```python
from build123d import *

# Parameters (mm, degrees)
SKETCH_3_W                = 201
SKETCH_3_H                = 142
EXTRUDE_2_DEPTH           = 5
SKETCH_4_W                = 171
SKETCH_4_H                = 112
CUT_EXTRUDE_1_DEPTH       = 2.5
SKETCH_5_W                = 50
SKETCH_5_H                = 20
CUT_EXTRUDE_6_DEPTH       = 15
SKETCH_6_R                = 1.2
CUT_EXTRUDE_7_DEPTH       = 3
CUT_EXTRUDE_8_REACH       = 215.23
HOLE_WIZARD_1_D           = 2.4
HOLE_WIZARD_1_CSINK_D     = 4.5
HOLE_WIZARD_1_CSINK_ANGLE = 90
FILLET_1_R                = 7


with BuildPart() as part:
    # 草图3 → 凸台-拉伸2 (new body)
    with BuildSketch(Plane.XY):
        Rectangle(SKETCH_3_W, SKETCH_3_H)
    extrude(amount=EXTRUDE_2_DEPTH)

    # 草图4 → 切除-拉伸1 (cut)
    with BuildSketch(Plane.XY):
        Rectangle(SKETCH_4_W, SKETCH_4_H)
    extrude(amount=CUT_EXTRUDE_1_DEPTH, mode=Mode.SUBTRACT)

    # 草图5 → 切除-拉伸6 (cut)
    with BuildSketch(Plane.XY):
        with Locations((0, -52)):
            Rectangle(SKETCH_5_W, SKETCH_5_H)
    extrude(amount=CUT_EXTRUDE_6_DEPTH, mode=Mode.SUBTRACT)

    # 草图6 → 切除-拉伸7 (cut)
    with BuildSketch(Plane(origin=(0, 0, 0), x_dir=(-1, 0, 0), z_dir=(0, 0, -1))):
        with Locations((-93, 63.5)):
            Circle(SKETCH_6_R)
        with Locations((93, 63.5)):
            Circle(SKETCH_6_R)
        with Locations((93, -63.5)):
            Circle(SKETCH_6_R)
        with Locations((-93, -63.5)):
            Circle(SKETCH_6_R)
    extrude(amount=-CUT_EXTRUDE_7_DEPTH, mode=Mode.SUBTRACT)

    # 草图9 → 切除-拉伸8 (cut, up to next)
    with BuildSketch(Plane.ZY.offset(100.5), mode=Mode.PRIVATE) as cut_extrude_8_sk1:
        Polygon((0, -71), (5, -71), (5, -68.113248654), align=None)
    cut_extrude_8_tool1 = extrude(cut_extrude_8_sk1.sketch, amount=-CUT_EXTRUDE_8_REACH, mode=Mode.PRIVATE) & part.part
    add(cut_extrude_8_tool1.solids().sort_by_distance((-100.5, -70.03775, 3.333333))[0], mode=Mode.SUBTRACT)

    # 打孔尺寸(%根据十字)槽沉头自攻螺钉的类型1 (through all)
    with Locations(Plane(origin=(0, 0, 0), x_dir=(-1, 0, 0), z_dir=(0, 0, -1))):
        with Locations((-93, -22.170448124), (-46.5, -63.5), (46.5, -63.5), (93, -22.170448124)):
            CounterSinkHole(HOLE_WIZARD_1_D / 2, HOLE_WIZARD_1_CSINK_D / 2, counter_sink_angle=HOLE_WIZARD_1_CSINK_ANGLE)

    # 圆角1
    fillet_1_edges = [part.edges().sort_by_distance(p)[0] for p in [
        (-100.5, 71, 2.5),
        (100.5, 71, 2.5),
    ]]
    fillet(fillet_1_edges, radius=FILLET_1_R)


solid = part.part
```
CAD build for the part. Positions are in the model's coordinates, mm. A direction names the side the tool comes from. Round coordinates to 2 decimals unless told otherwise and drop trailing zeros. Write each loop counter-clockwise with the first axis right and the second up, starting at its lowest first coordinate (ties: lowest second). Pieces come first, ordered by that corner, then holes. Notation, with made-up numbers: (0, 28.25) -> (40, 28.25) arc R28 ccw to (40, 61.25) -> close; hole circle Ø1 at (-14.5, 42.5). An arc over 180 degrees is marked (long way). Answer in a Markdown table with one row per item. Add a question column.
Item 1: Saw through at A-A, the plane y = -44. Write the cut outline in (x, z).
Item 2: Drill centre lines: line 1 (X direction, y = 55, z = 2.1); line 2 (Y direction, x = -93, z = 1); line 3 (Y direction, x = -93, z = 1.7). Where is each one in solid material? Low to high. Write a range as from..to.
Item 3: Drop flat-ended pins along their axis: pin 1 Ø1.2 at (x, y) = (-93.5, -63.5) entering from -Z; pin 2 Ø5 at (x, y) = (45.5, 5) entering from -Z; pin 3 Ø1.2 at (x, z) = (8, 3) entering from -Y. Give the stop position or say it passes through.
Item 4: Mould opens along X. For faces 4 (the face through (-100.5, -4, 2)), 5 (the face through (0, -62, 2)), 6 (the face through (-1, 2, 5)) say: pulls with the +X half, pulls with the -X half, needs draft (parallel to the pull), parting line crosses it, or undercut.
Item 5: Saw through at B-B, the plane x = 36.5. Write the cut outline in (y, z).
Item 6: Which spindle directions (+Z, -Z, +X, -X, +Y, -Y) get a long thin tool onto all of the face, cutting with end or side? Do faces 1 (the face through (-1.41, -69.54, 2.53)), 2 (the face through (25, -54, 3)), 3 (the face through (-1, 1, 2.5)). Say none if no direction does.
Item 7: Saw through at C-C, the plane y = 2.5. Write the cut outline in (x, z).
Findings below:
| question | item | result |
|---|---|---|
| 1 | outline | (-100.5, 0) -> (-85.5, 0) -> (-85.5, 2.5) -> (-25, 2.5) -> (-25, 5) -> (-100.5, 5) -> close; (25, 2.5) -> (85.5, 2.5) -> (85.5, 0) -> (100.5, 0) -> (100.5, 5) -> (25, 5) -> close |
| 2 | line 1 | x = -100.5..-85.5, 85.5..100.5 |
| 2 | line 2 | y = -70.42..-64.7, -62.3..-23.42, -20.92..62.3, 64.7..71 |
| 2 | line 3 | y = -70.02..-64.7, -62.3..-23.37, -20.97..62.3, 64.7..71 |
| 3 | pin 1 | stops at z = 3 |
| 3 | pin 2 | stops at z = 2.5 |
| 3 | pin 3 | stops at y = -69.61 |
| 4 | face 4 | pulls with the -X half |
| 4 | face 5 | undercut |
| 4 | face 6 | needs draft |
| 5 | outline | (-71, 0) -> (-56, 0) -> (-56, 2.5) -> (56, 2.5) -> (56, 0) -> (71, 0) -> (71, 5) -> (-68.11, 5) -> close |
| 6 | face 1 | +Z, +X, -X, -Y |
| 6 | face 2 | +Z, -Z |
| 6 | face 3 | -Z |
| 7 | outline | (-100.5, 0) -> (-85.5, 0) -> (-85.5, 2.5) -> (85.5, 2.5) -> (85.5, 0) -> (100.5, 0) -> (100.5, 5) -> (-100.5, 5) -> close |
